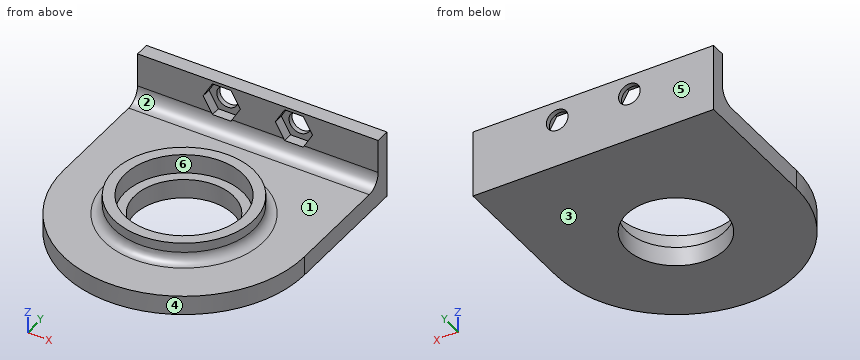
Autodesk Fusion 360 part; units mm, degrees
sketch "Esboço1" plane through (0, 0, 0) normal (0, 0, 1) x (1, 0, 0)
  line L0 (25, 28) -> (-25, 28)
  line L1 (-25, 0) -> (-25, 28)
  line L2 (25, 0) -> (25, 28)
  arc A0 (-25, 0) -> (25, 0) centre (0, 0) ccw
  circle A1 centre (0, 0) radius 10.25
  dimension "d1" = 50
  dimension "d3" = 28
  dimension "d4" = 20.5
extrude "Extrusão1" add sketch "Esboço1" along normal blind 4
sketch "Esboço2" plane through (0, 0, 4) normal (0, 0, 1) x (-1, 0, 0)
  circle A0 centre (0, 0) radius 10.25
  arc A1 (25, 0) -> (-25, 0) centre (0, 0) ccw
  line L0 (-25, 0) -> (-25, -28)
  line L1 (-25, -28) -> (25, -28)
  line L2 (25, -28) -> (25, 0)
  line L3 (25, -28) -> (-25, -28)
  line L4 (-25, -28) -> (-25, -25)
  line L5 (-25, -25) -> (25, -25)
  line L6 (25, -25) -> (25, -28)
  dimension "d7" = 3
extrude "Extrusão2" add sketch "Esboço2" along normal blind 10 contours L0 L1 L2 L3 L4 L5 L6
fillet "Arredondamento2" radius 3 1 edges at (0, 25, 4)
sketch "Esboço3" plane through (0, 28, 0) normal (0, 1, 0) x (-1, 0, 0)
  line L0 (-25, 0) -> (25, 0)
  line L1 (25, 0) -> (25, 14)
  line L2 (25, 14) -> (-25, 14)
  line L3 (-25, 14) -> (-25, 0)
  circle A0 centre (-7.5, 10) radius 2.25
  line L4 (0, -15) -> (0, 41) construction
  circle A1 centre (7.5, 10) radius 2.25
  dimension "d14" = 4.5
  dimension "d15" = 10
  dimension "d25" = 7.5
extrude "Extrusão3" cut sketch "Esboço3" against normal up to surface (3 mm away) contours A0 | A1
sketch "Esboço4" plane through (0, 0, 4) normal (0, 0, 1) x (-1, 0, 0)
  line L0 (-25, -22) -> (25, -22)
  line L1 (25, -22) -> (25, 0)
  arc A0 (25, 0) -> (-25, 0) centre (0, 0) ccw
  line L2 (-25, 0) -> (-25, -22)
  circle A1 centre (0, 0) radius 10.25
  circle A2 centre (0, 0) radius 12.25
  circle A3 centre (0, 0) radius 14.5
  dimension "d19" = 24.5
  dimension "d20" = 29
extrude "Extrusão4" add sketch "Esboço4" along normal blind 4 contours A3
fillet "Arredondamento3" radius 2 1 edges at (13.5187, -5.2434, 4)
sketch "Esboço5" plane through (0, 25, 0) normal (0, -1, 0) x (1, 0, 0)
  circle A0 centre (7.5, 10) radius 2.25
  circle A1 centre (-7.5, 10) radius 2.25
  line L0 (-25, 7) -> (25, 7)
  line L1 (25, 7) -> (25, 14)
  line L2 (25, 14) -> (-25, 14)
  line L3 (-25, 14) -> (-25, 7)
  line L4 (-5.566, 13.3498) -> (-9.434, 13.3498)
  line L5 (-9.434, 13.3498) -> (-11.368, 10)
  line L6 (-11.368, 10) -> (-9.434, 6.6502)
  line L7 (-9.434, 6.6502) -> (-5.566, 6.6502)
  line L8 (-5.566, 6.6502) -> (-3.632, 10)
  line L9 (-3.632, 10) -> (-5.566, 13.3498)
  line L10 (0, 0) -> (0, 14) construction
  line L11 (3.632, 10) -> (5.566, 13.3498)
  line L12 (5.566, 13.3498) -> (9.434, 13.3498)
  line L13 (9.434, 13.3498) -> (11.368, 10)
  line L14 (11.368, 10) -> (9.434, 6.6502)
  line L15 (9.434, 6.6502) -> (5.566, 6.6502)
  line L16 (5.566, 6.6502) -> (3.632, 10)
  point P0 (-7.5, 10)
  dimension "d26" = 7.736
extrude "Extrusão5" cut sketch "Esboço5" along normal mid plane 4 contours L0 L4 L5 L6 L8 L9 | L0 L6 L7 L8 | L0 L11 L12 L13 L14 L16 | L0 L14 L15 L16
equation "d8 = 7.75 mm + ( 4.5 / 2 ) * 1 mm"
equation "d15 = 7.75 mm + ( 4.5 / 2 ) * 1 mm"
equation "d25 = ( 15 / 2 ) * 1 mm"
Here's how the part is built. I have some questions about the finished solid (model axes, mm). Face numbers are marked on the shaded views. A direction names the side the tool comes from. Give positions to 0.01 mm unless a question says otherwise; leave off trailing zeros. Order: outer loops, then holes, each group sorted by start corner. A loop starts at its lowest first (then second) coordinate and runs counter-clockwise, first axis right, second up. Notation, with made-up numbers: (9, 85) -> (42, 85) arc R17 cw to (42, 99) -> close; hole circle Ø3 at (18.5, -34.75). An arc over 180 degrees is marked (long way). Use CSV: the item, a comma, the result in double quotes. Start each with the question number.
Item 1: Thinking about a two-plate mould opening in Y: for the marked faces 4, 5 and 6, which applies, pulls with the +Y half, pulls with the -Y half, needs draft (parallel to the pull), parting line crosses it, or undercut?
Item 2: Suppose I cut it at B-B (z = 11.25). List the corners of the cut face in (x, y) for me.
Item 3: If I drill on probe 1 along X at (y, z) = (27.4, 10); probe 2 along X at (y, z) = (0, 5.95); probe 3 along Y at (x, z) = (0, 5.9), over which ranges is the centre line in solid material (lowest first)? Write a range as [from, to].
Item 4: Suppose I cut it at A-A (x = 0). List the corners of the cut face in (y, z) for me.
Item 5: Suppose I cut it at C-C (x = 21). List the corners of the cut face in (y, z) for me.
Item 6: Suppose I cut it at D-D (x = 7.5). Give the number of separate pieces and of enclosed holes in the cut face, and give its area (3 significant figures).
Item 7: I'm going to push flat-ended pins straight in: P1, Ø12.5, axis at x = 0, y = 0, coming from the -Z side; P2, Ø2, axis at x = 3.5, y = 19.5, coming from the -Z side; P3, Ø2, axis at x = 9.5, z = 8.5, coming from the -Y side; P4, Ø2, axis at x = 17.5, y = 13, coming from the +Z side. Where does each tip first touch, or does it pass through?
Item 8: On a 3-axis mill with a long thin cutter (end or side, diameter ignored), from which of +Z, -Z, +X, -X, +Y, -Y can I reach the whole of each face in a straight line? I mean the marked faces 1, 2 and 3. Say none if no direction works.
Answer block:
1,face 4,"pulls with the -Y half"
1,face 5,"pulls with the +Y half"
1,face 6,"undercut"
2,outline,"(-25, 25) -> (-10.65, 25) -> (-10.65, 27) -> (-9.37, 27) -> (-9.37, 28) -> (-25, 28) -> close; (-5.63, 27) -> (-4.35, 27) -> (-4.35, 25) -> (4.35, 25) -> (4.35, 27) -> (5.63, 27) -> (5.63, 28) -> (-5.63, 28) -> close; (9.37, 27) -> (10.65, 27) -> (10.65, 25) -> (25, 25) -> (25, 28) -> (9.37, 28) -> close"
3,probe 1,"x = [-25, -9.75], [-5.25, 5.25], [9.75, 25]"
3,probe 2,"x = [-14.5, -12.25], [12.25, 14.5]"
3,probe 3,"y = [-14.5, -12.25], [12.25, 14.5], [24.79, 28]"
4,outline,"(-25, 0) -> (-10.25, 0) -> (-10.25, 4) -> (-12.25, 4) -> (-12.25, 8) -> (-14.5, 8) -> (-14.5, 6) arc R2 cw to (-16.5, 4) -> (-25, 4) -> close; (10.25, 0) -> (28, 0) -> (28, 14) -> (25, 14) -> (25, 7) arc R3 cw to (22, 4) -> (16.5, 4) arc R2 cw to (14.5, 6) -> (14.5, 8) -> (12.25, 8) -> (12.25, 4) -> (10.25, 4) -> close"
5,outline,"(-13.56, 0) -> (28, 0) -> (28, 14) -> (25, 14) -> (25, 7) arc R3 cw to (22, 4) -> (-13.56, 4) -> close"
6,separate pieces,"3"
6,enclosed holes,"0"
6,area,"189 mm^2"
7,P1,"passes through"
7,P2,"stops at z = 0"
7,P3,"stops at y = -11.65"
7,P4,"stops at z = 4"
8,face 1,"+Z"
8,face 2,"+Z, +X, -X"
8,face 3,"-Z, +X, -X, +Y, -Y"
